Build history of the part. All positions in model axes, mm. Give positions to 0.01 mm unless a question says otherwise; leave off trailing zeros. Write each loop counter-clockwise with the first axis right and the second up, starting at its lowest first coordinate (ties: lowest second). Pieces come first, ordered by that corner, then holes. Notation, with made-up numbers: (-28, 32.5) -> (0, 32.5) arc R31 cw to (0, 66.5) -> close; hole circle Ø2 at (2.25, -33.75). An arc over 180 degrees is marked (long way). Put each result on its own line as item: value.
from build123d import *

# Parameters (mm, degrees)
SKETCH2_W                      = 12.5
SKETCH2_H                      = 88
BOSS_EXTRUDE1_DEPTH            = 1.6
F_3_2_3_2_DIAMETER_HOLE1_D     = 3.2
F_3_2_3_2_DIAMETER_HOLE1_DEPTH = 1.6
F_3_2_3_2_DIAMETER_HOLE1_TIP   = 0.96137699
FILLET1_R                      = 3


with BuildPart() as part:
    # Sketch2 → Boss-Extrude1 (new body)
    with BuildSketch(Plane.XY.offset(96.838346843)):
        with Locations((-53.102520427, -5.981220417)):
            Rectangle(SKETCH2_W, SKETCH2_H)
    extrude(amount=BOSS_EXTRUDE1_DEPTH)

    # Ø3.2 (3.2) Diameter Hole1
    with Locations(Plane.XY.offset(98.438346843)):
        with Locations((-50.352520427, 29.018779583), (-50.352520427, -46.981220417)):
            Hole(F_3_2_3_2_DIAMETER_HOLE1_D / 2, depth=F_3_2_3_2_DIAMETER_HOLE1_DEPTH)
            with Locations((0, 0, -(F_3_2_3_2_DIAMETER_HOLE1_DEPTH + F_3_2_3_2_DIAMETER_HOLE1_TIP / 2))):  # 118° drill point
                Cone(0, F_3_2_3_2_DIAMETER_HOLE1_D / 2, F_3_2_3_2_DIAMETER_HOLE1_TIP, mode=Mode.SUBTRACT)

    # Fillet1
    fillet1_edges = [part.edges().sort_by_distance(p)[0] for p in [
        (-46.852520427, -49.981220417, 97.638346843),
        (-59.352520427, -49.981220417, 97.638346843),
        (-59.352520427, 38.018779583, 97.638346843),
        (-46.852520427, 38.018779583, 97.638346843),
    ]]
    fillet(fillet1_edges, radius=FILLET1_R)


solid = part.part
1) Pull direction Y, two halves, no side cores. Call faces 1 (the cylindrical face through (-58.497, 37.117, 97.65)), 2 (the cylindrical face through (-47.71, -49.08, 97.65)), 3 (the cylindrical face through (-51.09, 27.6, 97.63)), 4 (the flat face through (-59.353, -7, 98)): released by +Y, released by -Y, zero draft, split by the parting line, or undercut.
Filled sheet:
face 1: released by +Y
face 2: released by -Y
face 3: undercut
face 4: zero draft
2) Wall check: L1, parallel to Y at x = -50.25, z = 98.25; L2, parallel to Y at x = -50, z = 97.75; L3, parallel to X at y = 29, z = 98.35. Give the ranges that are in metal, low to high.
Filled sheet:
L1: -49.98 to -48.58, -45.38 to 27.42, 30.62 to 38.02
L2: -49.98 to -48.54, -45.42 to 27.46, 30.58 to 38.02
L3: -59.35 to -51.95, -48.75 to -46.85
3) Slice it at A-A (x = -51). Write the cut outline in (y, z), plus the area to 3 significant figures.
Filled sheet:
outline: (-49.98, 96.84) -> (-48.44, 96.84) -> (-48.44, 98.44) -> (-49.98, 98.44) -> close; (-45.52, 96.84) -> (27.56, 96.84) -> (27.56, 98.44) -> (-45.52, 98.44) -> close; (30.48, 96.84) -> (38.02, 96.84) -> (38.02, 98.44) -> (30.48, 98.44) -> close
area: 131 mm2
4) Slice it at B-B (z = 97.25). Write the cut outline in (x, y).
Filled sheet:
outline: (-59.35, -46.98) arc R3 ccw to (-56.35, -49.98) -> (-49.85, -49.98) arc R3 ccw to (-46.85, -46.98) -> (-46.85, 35.02) arc R3 ccw to (-49.85, 38.02) -> (-56.35, 38.02) arc R3 ccw to (-59.35, 35.02) -> close; hole circle Ø3.2 at (-50.35, -46.98); hole circle Ø3.2 at (-50.35, 29.02)
